Answer from the drawing. Dimensions are ordinates in mm from the lowest x, y and z of the part. A direction names the side the tool comes from. Give positions to 0.01 mm unless a question says otherwise; leave off trailing zeros. Order: outer loops, then holes, each group sorted by start corner. A loop starts at its lowest first (then second) coordinate and runs counter-clockwise, first axis right, second up. Notation, with made-up numbers: (-6, 15.5) -> (6, 15.5) arc R15 cw to (6, 26.5) -> close; hole circle Ø2 at (-25.5, 57). An arc over 180 degrees is marked (long way). Answer as a JSON object with one key per item and string values. Group by question number.
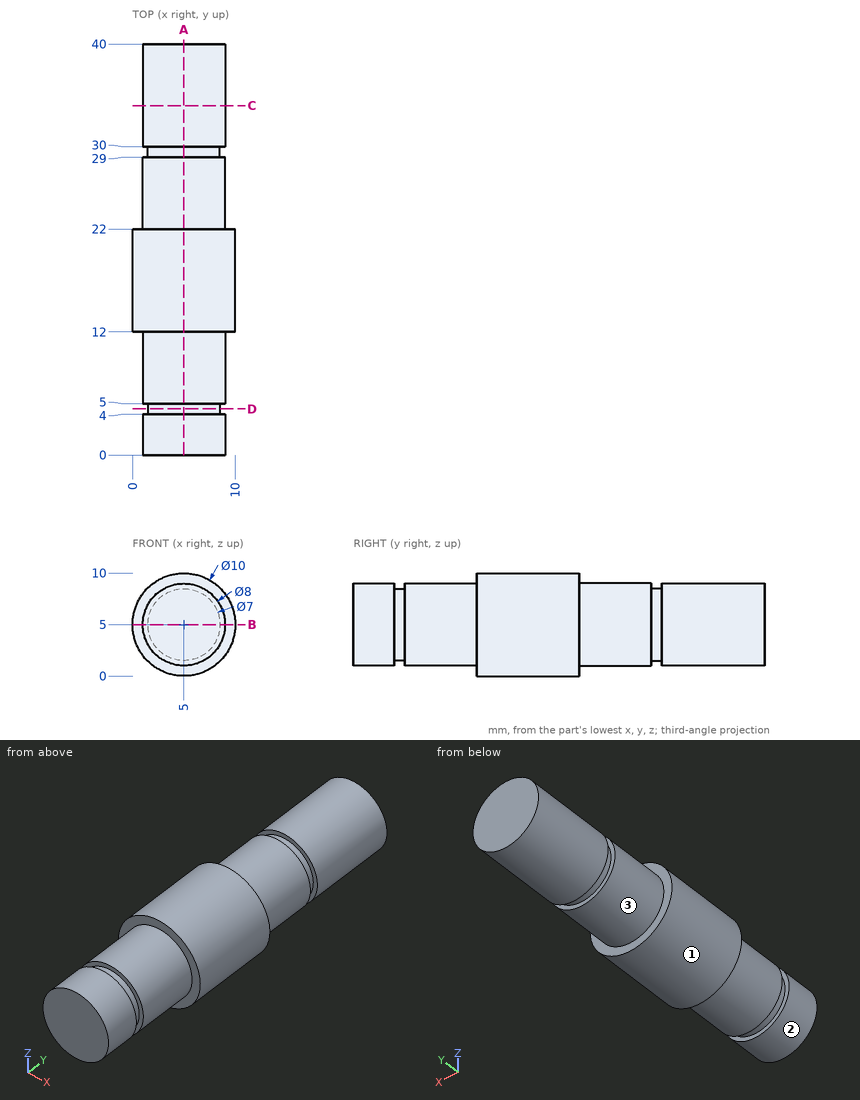
(1) A cutting plane is placed at C-C (y = 34). Determine the outline of the cut face in (x, z).
(2) Find the intervals of material crossed by line 1 along Y through (x, z) = (8, 8); line 2 along X through (y, z) = (38.5, 4.75), in increasing order. Write a range as [from, to].
(3) A cutting plane is placed at A-A (x = 5). Determine the outline of the cut face in (y, z).
(4) A cutting plane is placed at D-D (y = 4.5). Determine the outline of the cut face in (x, z), and give its area (3 significant figures).
(5) A cutting plane is placed at B-B (z = 5). Determine the outline of the cut face in (x, y).
(6) Flat-ended cylindrical pins translate along their axes: pin 1 Ø4 at (x, z) = (9, 7.5) entering from +Y; pin 2 Ø4 at (x, y) = (4, 6) entering from -Z; pin 3 Ø6 at (y, z) = (28.5, 3.5) entering from +X. Find the tip coordinate at first contact, or state that the pin passes through.
(7) Which of the six approach directions +Z, -Z, +X, -X, +Y, -Y give full straight-line access (tool end or side, diameter ignored) to the marked faces 1, 2 and 3?
Check sheet entries:
{
 "1": {"outline": "circle Ø8 at (5, 5)"},
 "2": {"line 1": "y = [12, 22]", "line 2": "x = [1.01, 8.99]"},
 "3": {"outline": "(0, 1) -> (4, 1) -> (4, 1.5) -> (5, 1.5) -> (5, 1) -> (12, 1) -> (12, 0) -> (22, 0) -> (22, 1) -> (29, 1) -> (29, 1.5) -> (30, 1.5) -> (30, 1) -> (40, 1) -> (40, 9) -> (30, 9) -> (30, 8.5) -> (29, 8.5) -> (29, 9) -> (22, 9) -> (22, 10) -> (12, 10) -> (12, 9) -> (5, 9) -> (5, 8.5) -> (4, 8.5) -> (4, 9) -> (0, 9) -> close"},
 "4": {"outline": "circle Ø7 at (5, 5)", "area": "38.5 mm2"},
 "5": {"outline": "(0, 12) -> (1, 12) -> (1, 5) -> (1.5, 5) -> (1.5, 4) -> (1, 4) -> (1, 0) -> (9, 0) -> (9, 4) -> (8.5, 4) -> (8.5, 5) -> (9, 5) -> (9, 12) -> (10, 12) -> (10, 22) -> (9, 22) -> (9, 29) -> (8.5, 29) -> (8.5, 30) -> (9, 30) -> (9, 40) -> (1, 40) -> (1, 30) -> (1.5, 30) -> (1.5, 29) -> (1, 29) -> (1, 22) -> (0, 22) -> close"},
 "6": {"pin 1": "stops at y = 40", "pin 2": "stops at z = 1", "pin 3": "stops at x = 9"},
 "7": {"face 1": "+Y, -Y", "face 2": "-Y", "face 3": "+Y"}
}
